Design review of the part built by this model. Coordinates are the model's own, in mm. A direction names the side the tool comes from. Round coordinates to 2 decimals unless told otherwise and drop trailing zeros. Write each loop counter-clockwise with the first axis right and the second up, starting at its lowest first coordinate (ties: lowest second). Pieces come first, ordered by that corner, then holes. Notation, with made-up numbers: M 69,0 L 74,0 A11 ccw 74,17 Z; hole C 2.25,76.25 d3. An arc over 180 degrees is marked long. One line per question, with ' | ' between items. Start each with the question number.
Item 1: Add section B-B, the plane z = 15.5. Give the number of separate pieces and of enclosed holes in the cut face, and give its area (3 significant figures).
Item 2: Add section A-A, the plane y = 113. State the section outline as (x, z) points, and give its area (3 significant figures).
Item 3: Insertion check: pin 1 Ø4 at (x, z) = (-161.5, 16.5) entering from +Y; pin 2 Ø3 at (x, y) = (-122.34, 100.1) entering from -Z; pin 3 Ø3 at (x, z) = (-163.5, 4) entering from +Y; pin 4 Ø5 at (x, z) = (-151.5, 3) entering from -Y. Each pin has a flat end and moves straight along its axis. Give the tip position at first contact, or say it passes through.
Item 4: Machinability: for faces 1 (the face through (-172.585, 154, 9)), 2 (the face through (-125, 175, 19.05)), which of the approach directions +Z, -Z, +X, -X, +Y, -Y give a long, thin tool a straight path to every point of the face, cutting with its end or side? Answer none if there is none.
Item 5: Add section C-C, the plane y = 220.5. State the section outline as (x, z) points.
Item 6: Draft analysis for pull direction Y (two halves, no side actions). For faces 3 (the face through (-174.265, 156.048, 9.658)), 4 (the face through (-176, 96.7, 10)), 5 (the face through (-122.7, 155.04, 9.66)), 6 (the face through (-125.585, 155, 9)), state which applies: released by +Y, released by -Y, zero draft, split by the parting line, or undercut.
Item 7: Add section D-D, the plane x = -166. State the section outline as (y, z) points.
Item 8: For L1, parallel to X at y = 117, z = 11.75; L2, parallel to X at y = 158, z = 17.75; L3, parallel to Y at x = -147, z = 7, list the stretches that pass through material, from the lowest coordinate up.
```python
from build123d import *

# Parameters (mm, degrees)
BOSS_EXTRUDE1_DEPTH = 19.05
SKETCH2_R           = 1.7
CUT_EXTRUDE1_DEPTH  = 20.05
CUT_EXTRUDE2_DEPTH  = 20.05


with BuildPart() as part:
    # Sketch1 → Boss-Extrude1 (new body)
    with BuildSketch(Plane.XY):
        with BuildLine():
            Line((-179.085368151, -18.789194183), (-179.085368151, 212.188334746))
            ThreePointArc((-179.085368151, 212.188334746), (-149.085368151, 242.188334746), (-119.085368151, 212.188334746))
            Line((-119.085368151, 212.188334746), (-119.085368151, -18.789194183))
            ThreePointArc((-119.085368151, -18.789194183), (-149.085368151, -48.789194183), (-179.085368151, -18.789194183))
        make_face()
        with BuildLine():
            Line((-172.585368151, -18.789194183), (-172.585368151, 212.188334746))
            ThreePointArc((-172.585368151, 212.188334746), (-149.085368151, 235.688334746), (-125.585368151, 212.188334746))
            Line((-125.585368151, 212.188334746), (-125.585368151, -18.789194183))
            ThreePointArc((-125.585368151, -18.789194183), (-149.085368151, -42.289194183), (-172.585368151, -18.789194183))
        make_face(mode=Mode.SUBTRACT)
    extrude(amount=BOSS_EXTRUDE1_DEPTH)

    # Sketch2 → Cut-Extrude1 (cut, through all)
    with BuildSketch(Plane.XY.offset(19.05)):
        with Locations((-145.785368151, 238.734002942)):
            Circle(SKETCH2_R)
        with Locations((-122.335368151, 212.188334746)):
            Circle(SKETCH2_R)
        with Locations((-152.485368151, -45.322239617)):
            Circle(SKETCH2_R)
        with Locations((-168.000474547, -37.70430058)):
            Circle(SKETCH2_R)
        with Locations((-175.835368151, -18.789194183)):
            Circle(SKETCH2_R)
        with Locations((-175.835368151, 212.188334746)):
            Circle(SKETCH2_R)
        with Locations((-145.685368151, -45.322239617)):
            Circle(SKETCH2_R)
        with Locations((-175.835368151, 100.099570281)):
            Circle(SKETCH2_R)
        with Locations((-175.835368151, 93.299570281)):
            Circle(SKETCH2_R)
        with Locations((-122.335368151, 100.099570281)):
            Circle(SKETCH2_R)
        with Locations((-122.335368151, 93.299570281)):
            Circle(SKETCH2_R)
        with Locations((-122.335368151, -18.789194183)):
            Circle(SKETCH2_R)
        with Locations((-130.170261754, -37.70430058)):
            Circle(SKETCH2_R)
        with Locations((-175.835368151, 156.699570281)):
            Circle(SKETCH2_R)
        with Locations((-122.335368151, 156.699570281)):
            Circle(SKETCH2_R)
        with Locations((-175.835368151, 66.699570281)):
            Circle(SKETCH2_R)
        with Locations((-122.335368151, 66.699570281)):
            Circle(SKETCH2_R)
        with Locations((-175.835368151, 36.699570281)):
            Circle(SKETCH2_R)
        with Locations((-122.335368151, 36.699570281)):
            Circle(SKETCH2_R)
        with Locations((-175.835368151, 6.699570281)):
            Circle(SKETCH2_R)
        with Locations((-122.335368151, 6.699570281)):
            Circle(SKETCH2_R)
        with Locations((-152.385368151, 238.734002942)):
            Circle(SKETCH2_R)
    extrude(amount=-CUT_EXTRUDE1_DEPTH, mode=Mode.SUBTRACT)

    # Sketch3 → Cut-Extrude2 (cut, through all)
    with BuildSketch(Plane.XY.offset(19.05)):
        Polygon((-149.085368151, 96.699570281), (-100.167336626, 96.699570281), (-100.167336626, -59.171887956), (-212.527814826, -59.171887956), (-212.527814826, 96.699570281), align=None)
    extrude(amount=-CUT_EXTRUDE2_DEPTH, mode=Mode.SUBTRACT)


solid = part.part
```
Computed values:
1) separate pieces: 1 | enclosed holes: 8 | area: 1,970 mm^2
2) outline: M -179.09,0 L -172.59,0 L -172.59,19.05 L -179.09,19.05 Z; M -125.59,0 L -119.09,0 L -119.09,19.05 L -125.59,19.05 Z | area: 248 mm^2
3) pin 1: stops at y = 240.32 | pin 2: passes through | pin 3: stops at y = 239.27 | pin 4: stops at y = 235.17
4) face 1: +Z, -Z, -Y | face 2: +Z, +X, -X, +Y, -Y
5) outline: M -177.91,0 L -171.07,0 L -171.07,19.05 L -177.91,19.05 Z; M -127.1,0 L -120.26,0 L -120.26,19.05 L -127.1,19.05 Z
6) face 3: undercut | face 4: released by -Y | face 5: undercut | face 6: zero draft
7) outline: M 228.5,0 L 236.97,0 L 236.97,19.05 L 228.5,19.05 Z
8) L1: x = -179.09 to -172.59, -125.59 to -119.09 | L2: x = -179.09 to -176.93, -174.74 to -172.59, -125.59 to -123.43, -121.24 to -119.09 | L3: y = 235.6 to 237.54, 239.92 to 242.12
